The listing builds one solid part. Answer for the finished solid, in the listing's coordinates (mm). A direction names the side the tool comes from. Give positions to 0.01 mm unless a question says otherwise; leave off trailing zeros. Write each loop counter-clockwise with the first axis right and the second up, starting at its lowest first coordinate (ties: lowest second). Pieces come first, ordered by that corner, then holes. Notation, with made-up numbers: (-11.5, -2) - (13.5, -2) arc R9 ccw to (13.5, 15) - close; hole circle Ø5 at (58, 46.25). An arc over 180 degrees is marked (long way). One line per question, with ' | ' between items. Start each with the question number.
1. The mould has two halves that part along Z. Classify faces 4 (the face through (2, -4, -7.5)), 5 (the face through (7.49, -31.93, -0.65)), 6 (the face through (4, -25, 7.5)), 7 (the face through (2.172, -36.551, 6.702)): +Z half, -Z half, draft (parallel to the pull), parting line (faces both ways), or undercut.
2. A cutting plane is placed at A-A (y = -3.5). Determine the outline of the cut face in (x, z).
3. Given P1, Ø1, axis at x = 6, z = -4.5, coming from the +Y side; P2, Ø4.5, axis at x = 2, y = -15.5, coming from the -Z side; P3, Ø2.5, axis at x = 3.5, z = 1, coming from the -Y side, each flat-ended and moving along its own axis, determine where each tip first touches the part or whether it passes through.
4. A cutting plane is placed at B-B (y = -37). Determine the outline of the cut face in (x, z).
5. Find the intervals of material crossed by L1, parallel to Y at x = 7, z = 0; L2, parallel to Y at x = 7, z = -1.5; L3, parallel to Y at x = 2.35, z = 3.5, in increasing order. Write a range as from..to.
6. A cutting plane is placed at D-D (x = 8). Determine the outline of the cut face in (y, z), then the cut area to 3 significant figures.
7. For faces 1 (the face through (2, -10, -5)), 2 (the face through (5.4, -20, -0.5)), 3 (the face through (3, -24, 0)), determine the directions among +Z, -Z, +X, -X, +Y, -Y from which every point of the face is accessible in a straight line to the end or side of a thin tool.
8. A cutting plane is placed at C-C (z = 0.75). Determine the outline of the cut face in (x, y).
```python
from build123d import *

# Parameters (mm, degrees)
DODANIE_WYCI_GNI_CIE1_DEPTH = 7.5
SZKIC2_W                    = 6.5
SZKIC2_H                    = 11
WYTNIJ_WYCI_GNI_CIE1_DEPTH  = 26
WYTNIJ_WYCI_GNI_CIE2_REACH  = 53.269
SZKIC4_R                    = 1.6
SZKIC4_R_2                  = 3
WYTNIJ_WYCI_GNI_CIE3_DEPTH  = 52.268898954
ZAOKR_GLENIE1_R             = 3
ZAOKR_GLENIE2_R             = 1.5
SFAZOWANIE2_SIZE            = 1
SFAZOWANIE3_SIZE            = 2


with BuildPart() as part:
    # Szkic1 → Dodanie-wyciągnięcie1 (new, symmetric)
    with BuildSketch(Plane.XY):
        Polygon((0, 0), (4, 0), (4, -20), (8.5, -20), (8.5, -50), (4.5, -50), (0, -24), align=None)
    extrude(amount=DODANIE_WYCI_GNI_CIE1_DEPTH, both=True)

    # Szkic2 → Wytnij-wyciągnięcie1 (cut)
    with BuildSketch(Plane.XZ.offset(50)):
        with Locations((3.25, 0)):
            Rectangle(SZKIC2_W, SZKIC2_H)
    extrude(amount=-WYTNIJ_WYCI_GNI_CIE1_DEPTH, mode=Mode.SUBTRACT)

    # Szkic3 → Wytnij-wyciągnięcie2 (cut, up to next)
    with BuildSketch(Plane.ZY, mode=Mode.PRIVATE) as wytnij_wyci_gni_cie2_sk1:
        Polygon((-7.5, -7.5), (-7.5, -20), (-2.5, -20), (-2.5, -12.5), align=None)
    wytnij_wyci_gni_cie2_tool1 = extrude(wytnij_wyci_gni_cie2_sk1.sketch, amount=-WYTNIJ_WYCI_GNI_CIE2_REACH, mode=Mode.PRIVATE) & part.part
    add(wytnij_wyci_gni_cie2_tool1.solids().sort_by_distance((0, -14.895833, -5.208333))[0], mode=Mode.SUBTRACT)

    # Szkic4 → Wytnij-wyciągnięcie3 (cut, through all)
    with BuildSketch(Plane.ZY):
        with Locations((-3.5, -3.5)):
            Circle(SZKIC4_R)
        with Locations((3.5, -3.5)):
            Circle(SZKIC4_R)
        with Locations((0, -29)):
            Circle(SZKIC4_R_2)
        with Locations((0, -37)):
            Circle(SZKIC4_R_2)
        with Locations((0, -45)):
            Circle(SZKIC4_R_2)
        with Locations((3.5, -10.5)):
            Circle(SZKIC4_R)
    extrude(amount=-WYTNIJ_WYCI_GNI_CIE3_DEPTH, mode=Mode.SUBTRACT)

    # Zaokrąglenie1
    zaokr_glenie1_edges = [part.edges().sort_by_distance(p)[0] for p in [
        (3.25, -24, -5.5),
        (3.25, -24, 5.5),
    ]]
    fillet(zaokr_glenie1_edges, radius=ZAOKR_GLENIE1_R)

    # Zaokrąglenie2
    zaokr_glenie2_edges = [part.edges().sort_by_distance(p)[0] for p in [
        (4.5, -50, 6.5),
        (4.5, -50, -6.5),
    ]]
    fillet(zaokr_glenie2_edges, radius=ZAOKR_GLENIE2_R)

    # Sfazowanie2
    sfazowanie2_edges = [part.edges().sort_by_distance(p)[0] for p in [
        (4, -20, 2.5),
        (8.5, -20, 0),
        (2, -20, -2.5),
    ]]
    chamfer(sfazowanie2_edges, length=SFAZOWANIE2_SIZE)

    # Sfazowanie3
    sfazowanie3_edges = [part.edges().sort_by_distance(p)[0] for p in [
        (3.75, -20, -7.5),
    ]]
    chamfer(sfazowanie3_edges, length=SFAZOWANIE3_SIZE)


solid = part.part
```
Determined:
1) face 4: -Z half | face 5: undercut | face 6: +Z half | face 7: draft
2) outline: (0, -7.5) - (4, -7.5) - (4, -5.1) - (0, -5.1) - close; (0, -1.9) - (4, -1.9) - (4, 1.9) - (0, 1.9) - close; (0, 5.1) - (4, 5.1) - (4, 7.5) - (0, 7.5) - close
3) P1: y = -20 | P2: z = -2.5 | P3: y = -24
4) outline: (2.25, -7.5) - (8.5, -7.5) - (8.5, -3) - (6.5, -3) - (6.5, -5.5) - (2.25, -5.5) - close; (2.25, 5.5) - (6.5, 5.5) - (6.5, 3) - (8.5, 3) - (8.5, 7.5) - (2.25, 7.5) - close
5) L1: -50..-48, -42..-40, -34..-32, -26..-20 | L2: -50..-47.6, -42.4..-39.6, -34.4..-31.6, -26.4..-20 | L3: -24.17..-12.1, -8.9..-5.1, -1.9..0
6) outline: (-50, -7.5) - (-22, -7.5) - (-20.5, -6) - (-20.5, 7.5) - (-50, 7.5) - close; hole circle Ø6 at (-45, 0); hole circle Ø6 at (-37, 0); hole circle Ø6 at (-29, 0) | area: 357 mm2
7) face 1: -Z, +X, -X | face 2: -Z, +X | face 3: -X, -Y
8) outline: (0, -24) - (6.5, -24) - (6.5, -26.1) - (8.5, -26.1) - (8.5, -21) - (7.5, -20) - (5, -20) - (4, -19) - (4, 0) - (0, 0) - close; (6.5, -50) - (8.5, -50) - (8.5, -47.9) - (6.5, -47.9) - close; (6.5, -42.1) - (8.5, -42.1) - (8.5, -39.9) - (6.5, -39.9) - close; (6.5, -34.1) - (8.5, -34.1) - (8.5, -31.9) - (6.5, -31.9) - close
